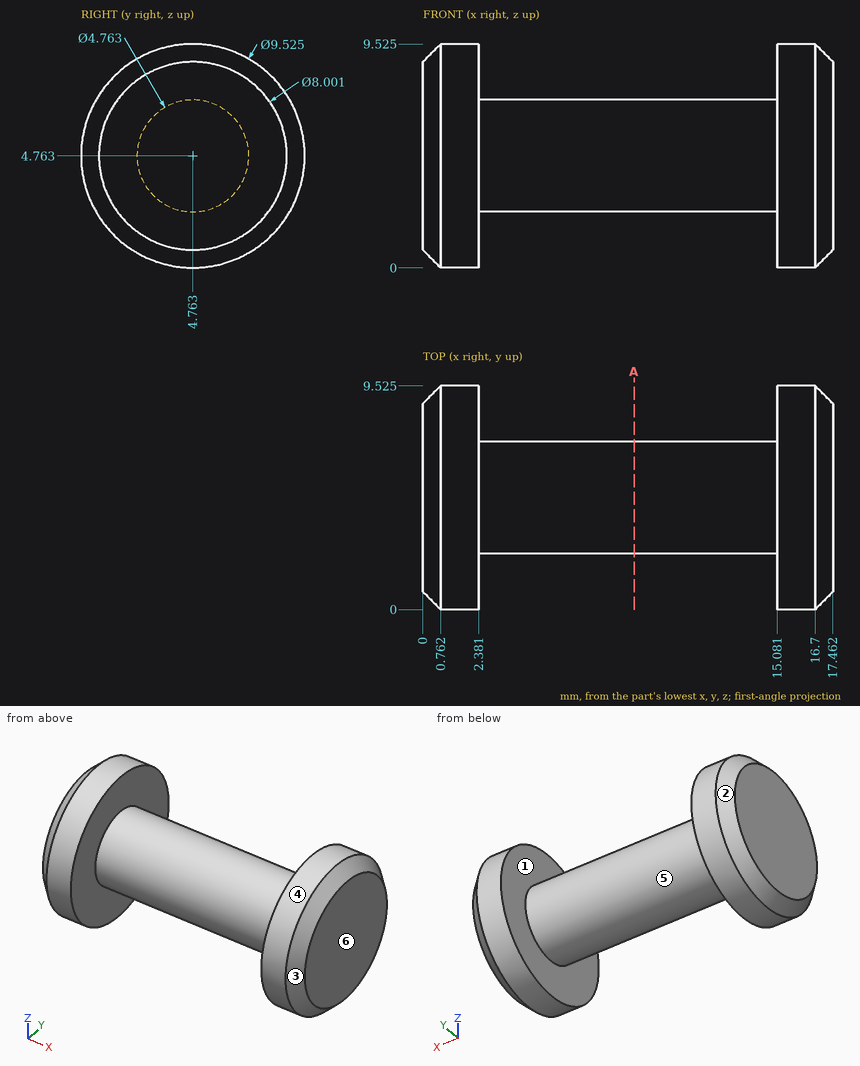
For this review, use the dimensioned drawing (mm, ordinates from the lowest corner) and the shaded views. A direction names the side the tool comes from. Give positions to 0.01 mm unless a question says otherwise; leave off trailing zeros. Order: outer loops, then holes, each group sorted by start corner. A loop starts at its lowest first (then second) coordinate and runs counter-clockwise, first axis right, second up.
1) For the marked faces 5 and 6, list the 3-axis set-ups (+Z, -Z, +X, -X, +Y, -Y) from which the entire face can be reached by the end or side of a thin tool; tool diameter is ignored.
2) Take a section at A-A (x = 9). Give the boundary of the cut face in (y, z).
3) The part is to be moulded in two halves that separate along X. For the marked faces 1, 2, 3 and 4, say which applies: released by +X, released by -X, zero draft, split by the parting line, or undercut.
4) Wall thickness on line 1 (X direction, y = 4, z = 1.5); line 2 (X direction, y = 1.75, z = 1.25) (1 decimal); line 3 (Y direction, x = 4, z = 3) (1 decimal): over which ranges is each line inside the solid? List them lowest first.
5) Insertion check: pin 1 (5 mm diameter, centred on x = 3.5, z = 6.5, fed in from -Y); pin 2 (4 mm diameter, centred on x = 6, y = 3.5, fed in from +Z); pin 3 (1 mm diameter, centred on x = 14.5, z = 5, fed in from -Y). Each pin has a flat end and moves straight along its axis. Give the tip position at first contact, or say it passes through.
Derived:
1. face 5: none
1. face 6: +Z, -Z, +X, +Y, -Y
2. outline: circle Ø4.76 at (4.76, 4.76)
3. face 1: undercut
3. face 2: released by -X
3. face 3: released by +X
3. face 4: zero draft
4. line 1: x = 0 to 2.38, 15.08 to 17.46
4. line 2: x = 0.6 to 2.4, 15.1 to 16.8
4. line 3: y = 3.2 to 6.4
5. pin 1: stops at y = 0
5. pin 2: stops at z = 7.14
5. pin 3: stops at y = 2.38
